Design review of the part built by this model. Coordinates are the model's own, in mm. Face numbers are marked on the shaded views. Give positions to 0.01 mm unless a question says otherwise; leave off trailing zeros. Write each loop counter-clockwise with the first axis right and the second up, starting at its lowest first coordinate (ties: lowest second). Pieces come first, ordered by that corner, then holes. Notation, with made-up numbers: M -18,-17.5 L 16,-17.5 A22 cw 16,0.5 Z; hole C 17,8.25 d3. An arc over 180 degrees is marked long. Answer in a Markdown table with one row per item.
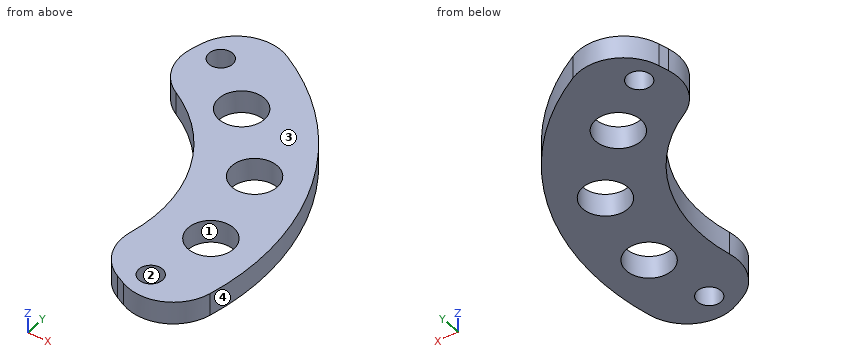
Autodesk Inventor part; units mm, degrees
ref_plane "YZ Plane" through (0, 0, 0) normal (1, 0, 0) x (0, 1, 0)
ref_plane "XZ Plane" through (0, 0, 0) normal (0, 1, 0) x (-1, 0, 0)
ref_plane "XY Plane" through (0, 0, 0) normal (0, 0, 1) x (1, 0, 0)
sketch "Sketch2" plane through (0, 0, 0) normal (0, 0, 1) x (1, 0, 0)
  circle A0 centre (28.194, 0) radius 3.175
  circle A1 centre (25.645, 11.7147) radius 3.175
  circle A2 centre (17.397, 20.4153) radius 3.175
  line L0 (0, 0) -> (28.194, 0) construction
  line L1 (25.645, 11.7147) -> (0, 0) construction
  line L2 (17.397, 20.4153) -> (0, 0) construction
  line L3 (18.663, -9.1026) -> (31.2762, -15.2544)
  line L4 (5.1766, 20.1089) -> (8.6751, 33.6993)
  arc A3 (18.663, -9.1026) -> (5.1766, 20.1089) centre (0, 0) ccw
  arc A4 (31.2762, -15.2544) -> (8.6751, 33.6993) centre (0, 0) ccw
  circle A5 centre (10.2574, 26.1255) radius 1.651
  circle A6 centre (26.5379, -9.1377) radius 1.651
  line L5 (10.2574, 26.1255) -> (0, 0) construction
  line L6 (0, 0) -> (26.5379, -9.1377) construction
  dimension "d2" = 6.35
  dimension "d4" = 28.194
  dimension "d5" = 26.8224
  dimension "d6" = 11.9888
  dimension "d7" = 11.9888
  dimension "d9" = 41.529
  dimension "d11" = 69.596
  dimension "d14" = 28.067
  dimension "d15" = 19
  dimension "d16" = 19
  dimension "d17" = 7
  dimension "d18" = 7
  dimension "d19" = 3.302
extrude "Extrusion1" add sketch "Sketch2" along normal blind 3.175
fillet "Fillet1" radius 6.35 4 edges at (8.6751, 33.6993, 1.5875) (5.1766, 20.1089, 1.5875) (18.663, -9.1026, 1.5875) (31.2762, -15.2544, 1.5875)
properties part number "gearboxBearingHolderForward" material "Aluminum 6061"
1) Add section B-B (x = 29.25). Write out the cut boundary in (y, z) (3 decimals).
Geometry says:
| item | result |
|---|---|
| outline | M -12.609,0 L -2.994,0 L -2.994,3.175 L -12.609,3.175 Z; M 2.994,0 L 18.85,0 L 18.85,3.175 L 2.994,3.175 Z |
2) To check wall thickness, follow probe 1 along Y at (x, z) = (26.5, 1); probe 2 along Y at (x, z) = (27.25, 1.1); probe 3 along X at (y, z) = (-8, 2.9) (3 decimals). State the ranges of each line that lie inside material, in increasing order. Write a range as [from, to].
Geometry says:
| item | result |
|---|---|
| probe 1 | [-12.68, -10.79], [-7.49, -2.69], [2.69, 8.66], [14.77, 22.55] |
| probe 2 | [-12.78, -10.63], [-7.65, -3.03], [3.03, 8.98], [14.45, 21.64] |
| probe 3 | [20.502, 25.341], [27.734, 33.865] |
3) Add section D-D (x = 25.5). Write out the cut boundary in (y, z) (3 decimals).
Geometry says:
| item | result |
|---|---|
| outline | M -12.403,0 L -10.422,0 L -10.422,3.175 L -12.403,3.175 Z; M -7.854,0 L -1.68,0 L -1.68,3.175 L -7.854,3.175 Z; M 1.68,0 L 8.543,0 L 8.543,3.175 L 1.68,3.175 Z; M 14.886,0 L 23.678,0 L 23.678,3.175 L 14.886,3.175 Z |
4) Insertion check: P1, Ø2, axis at x = 30, y = 14, coming from the -Z side; P2, Ø1, axis at x = 32, z = 0.5, coming from the -Y side. Each pin has a flat end and moves straight along its axis. Give the tip position at first contact, or say it passes through.
Geometry says:
| item | result |
|---|---|
| P1 | z = 0 |
| P2 | y = -11.54 |
5) The part is to be moulded in two halves that separate along Y. For the marked faces 1, 2, 3 and 4, say which applies: released by +Y, released by -Y, zero draft, split by the parting line, or undercut.
Geometry says:
| item | result |
|---|---|
| face 1 | undercut |
| face 2 | undercut |
| face 3 | zero draft |
| face 4 | split by the parting line |
6) Add section C-C (z = 0.6). Count the separate pieces of the cut face and the enclosed holes in it, and give its area (3 significant figures).
Geometry says:
| item | result |
|---|---|
| separate pieces | 1 |
| enclosed holes | 5 |
| area | 543 mm^2 |
7) Add section A-A (y = 0). Write out the cut boundary in (x, z) (1 decimal), and give its area (3 significant figures).
Geometry says:
| item | result |
|---|---|
| outline | M 20.8,0 L 25,0 L 25,3.2 L 20.8,3.2 Z; M 31.4,0 L 34.8,0 L 34.8,3.2 L 31.4,3.2 Z |
| area | 24.4 mm^2 |
